Read the model definition and answer for the solid it produces. Units are mm, in the model's axes. A direction names the side the tool comes from. Coordinates: 2 decimals unless noted, no trailing zeros. Loops run counter-clockwise (first coordinate to the right, second up) from the corner with the lowest first, then second, coordinate; pieces in that order, holes last.
from build123d import *

# Parameters (mm, degrees)
F0_W     = 76.2
F0_H     = 50.8
F0_R     = 12.7
F1_DEPTH = 12.7
F2_W     = 6.35
F2_H     = 50.8
F3_DEPTH = 2.54
F4_R     = 3.776277
F5_DEPTH = 18.542
F7_DEPTH = 50.801


with BuildPart() as f1:
    # F0 (on Top) → F1 (new body)
    with BuildSketch(Plane.XY):
        Rectangle(F0_W, F0_H)
        Circle(F0_R, mode=Mode.SUBTRACT)
    extrude(amount=F1_DEPTH)

    # F2 (on face) → F3 (cut)
    with BuildSketch(Plane.XY.offset(12.7)):
        with Locations((-32.385, 0)):
            Rectangle(F2_W, F2_H)
        with BuildLine():
            Line((-5.251254, -11.563491), (-5.251254, -25.4))
            Line((-5.251254, -25.4), (0, -25.4))
            Line((0, -25.4), (0, -12.7))
            ThreePointArc((0, -12.7), (-2.686416, -12.412621), (-5.251254, -11.563491))
        make_face()
        with BuildLine():
            Line((0, -12.7), (0, -25.4))
            Line((0, -25.4), (4.908746, -25.4))
            Line((4.908746, -25.4), (4.908746, -11.712993))
            ThreePointArc((4.908746, -11.712993), (2.503496, -12.450803), (0, -12.7))
        make_face()
        with BuildLine():
            Line((0, 25.4), (-5.251254, 25.4))
            Line((-5.251254, 25.4), (-5.251254, 11.563491))
            ThreePointArc((-5.251254, 11.563491), (-2.686416, 12.412621), (0, 12.7))
            Line((0, 12.7), (0, 25.4))
        make_face()
        with BuildLine():
            Line((4.908746, 25.4), (0, 25.4))
            Line((0, 25.4), (0, 12.7))
            ThreePointArc((0, 12.7), (2.503496, 12.450803), (4.908746, 11.712993))
            Line((4.908746, 11.712993), (4.908746, 25.4))
        make_face()
    extrude(amount=-F3_DEPTH, mode=Mode.SUBTRACT)

    # F4 (on face) → F5 (join)
    with BuildSketch(Plane.YZ.offset(38.1)):
        with Locations((0, 6.044753)):
            Circle(F4_R)
    extrude(amount=F5_DEPTH)

    # F6 (on face) → F7 (cut, through all)
    with BuildSketch(Plane.XZ.offset(25.4)):
        Polygon((26.256265, 12.7), (14.608031, 12.7), (12.698486, 7.924618), (28.356764, 7.924618), align=None)
    extrude(amount=-F7_DEPTH, mode=Mode.SUBTRACT)


solid = f1.part
Q1. Flat-ended cylindrical pins translate along their axes: pin 1 Ø0.8 at (y, z) = (-21, 11) entering from +X; pin 2 Ø5 at (x, y) = (-31.5, 11) entering from +Z; pin 3 Ø4.5 at (x, y) = (20.5, 9.5) entering from +Z; pin 4 Ø5 at (x, y) = (0, 20.5) entering from +Z. Find the tip coordinate at first contact, or state that the pin passes through.
Findings below:
pin 1: stops at x = 38.1
pin 2: stops at z = 12.7
pin 3: stops at z = 7.92
pin 4: stops at z = 10.16
Q2. Which of the six approach directions +Z, -Z, +X, -X, +Y, -Y give full straight-line access (tool end or side, diameter ignored) to faces 5 (the face through (-35.56, 0, 11)), 6 (the face through (20, 0, 7.925)), 7 (the face through (8, 12, 0))?
Findings below:
face 5: +Z, +Y, -Y
face 6: +Y, -Y
face 7: -Z, +X, -X, +Y, -Y
Q3. Determine the mould class of faces 1 (the face through (27.32, -0.36, 10.28)), 2 (the face through (13.67, -0.36, 10.35)), 3 (the face through (-38.1, 0, 6)), 4 (the face through (47.24, -0.82, 2.36)) for opening direction X: +X half, -X half, draft (parallel to the pull), parting line (faces both ways), or undercut.
Findings below:
face 1: undercut
face 2: undercut
face 3: -X half
face 4: draft
Q4. A cutting plane is placed at C-C (y = -15.5). Give the vertices of the cut face in (x, z).
Findings below:
outline: (-38.1, 0) - (38.1, 0) - (38.1, 12.7) - (26.26, 12.7) - (28.36, 7.92) - (12.7, 7.92) - (14.61, 12.7) - (4.91, 12.7) - (4.91, 10.16) - (-5.25, 10.16) - (-5.25, 12.7) - (-29.21, 12.7) - (-29.21, 10.16) - (-35.56, 10.16) - (-35.56, 12.7) - (-38.1, 12.7) - close
Q5. A cutting plane is placed at B-B (y = -2.5). Give the vertices of the cut face in (x, z) (1 decimal), then the cut area to 3 significant figures.
Findings below:
outline: (-38.1, 0) - (-12.5, 0) - (-12.5, 12.7) - (-29.2, 12.7) - (-29.2, 10.2) - (-35.6, 10.2) - (-35.6, 12.7) - (-38.1, 12.7) - close; (12.5, 0) - (38.1, 0) - (38.1, 3.2) - (56.6, 3.2) - (56.6, 8.9) - (38.1, 8.9) - (38.1, 12.7) - (26.3, 12.7) - (28.4, 7.9) - (12.7, 7.9) - (14.6, 12.7) - (12.5, 12.7) - close
area: 675 mm2
Q6. A cutting plane is placed at A-A (x = 0). Give the vertices of the cut face in (y, z), then the cut area to 3 significant figures.
Findings below:
outline: (-25.4, 0) - (-12.7, 0) - (-12.7, 10.16) - (-25.4, 10.16) - close; (12.7, 0) - (25.4, 0) - (25.4, 10.16) - (12.7, 10.16) - close
area: 258 mm2
Q7. A cutting plane is placed at D-D (y = -8). Give the vertices of the cut face in (x, z).
Findings below:
outline: (-38.1, 0) - (-9.86, 0) - (-9.86, 12.7) - (-29.21, 12.7) - (-29.21, 10.16) - (-35.56, 10.16) - (-35.56, 12.7) - (-38.1, 12.7) - close; (9.86, 0) - (38.1, 0) - (38.1, 12.7) - (26.26, 12.7) - (28.36, 7.92) - (12.7, 7.92) - (14.61, 12.7) - (9.86, 12.7) - close
Q8. Straight lines are drawn through the part: probe 1 along X at (y, z) = (0, 6); probe 2 along Y at (x, z) = (0, 4.25); probe 3 along X at (y, z) = (-20, 10.25). For each, find the intervals that lie inside material, in ascending order.
Findings below:
probe 1: x = -38.1 to -12.7, 12.7 to 56.64
probe 2: y = -25.4 to -12.7, 12.7 to 25.4
probe 3: x = -38.1 to -35.56, -29.21 to -5.25, 4.91 to 13.63, 27.33 to 38.1
